Here's how the part is built. I have some questions about the finished solid (model axes, mm). Round coordinates to 2 decimals unless told otherwise and drop trailing zeros. Write each loop counter-clockwise with the first axis right and the second up, starting at its lowest first coordinate (ties: lowest second). Pieces come first, ordered by that corner, then holes. Notation, with made-up numbers: (69, 1) - (102, 1) arc R9 ccw to (102, 15) - close; hole circle Ø1 at (60, -4.5). An arc over 180 degrees is marked (long way). One line per item, written item: value. Start each with the question number.
Item 1: Imagine slicing it at C-C, the plane y = -20. Please give me the cut outline in (x, z), then the cut area to 3 significant figures.
Item 2: Imagine slicing it at B-B, the plane x = 8.5. Please give me the cut outline in (y, z), then the cut area to 3 significant figures.
Item 3: If I drill on line 1 (X direction, y = 63.5, z = -0.1); line 2 (Y direction, x = -1, z = 0.1); line 3 (X direction, y = 31, z = 0.55), over which ranges is the centre line in solid material (lowest first)?
Item 4: Imagine slicing it at A-A, the plane z = 0. Please give me the cut outline in (x, y), then the cut area to 3 significant figures.
Item 5: For P1, Ø1.5, axis at x = 14.5, y = 19, coming from the -Z side; P2, Ø1, axis at x = 0.5, z = 1, coming from the -Y side, each with a flat end and sliding along its axis, tell me the tip position at first contact or that it passes through.
```python
from build123d import *

# Parameters (mm, degrees)
SKETCH5_R = 1.5


with BuildPart() as part:
    # Sweep2: sweep along a path in Sketch4
    with BuildLine(Plane.XY) as sweep2_path:
        Line((-23.236021708, 65.358068893), (-23.236021708, -37.641931107))
        ThreePointArc((-23.236021708, -37.641931107), (-18.549730207, -48.955639606), (-7.236021708, -53.641931107))
        Line((-7.236021708, -53.641931107), (12.563978292, -53.641931107))
        ThreePointArc((12.563978292, -53.641931107), (16.806618979, -51.884571794), (18.563978292, -47.641931107))
        Line((18.563978292, -47.641931107), (18.563978292, 65.358068893))
        ThreePointArc((18.563978292, 65.358068893), (16.806618979, 69.60070958), (12.563978292, 71.358068893))
        Line((12.563978292, 71.358068893), (-17.236021708, 71.358068893))
        ThreePointArc((-17.236021708, 71.358068893), (-21.478662395, 69.60070958), (-23.236021708, 65.358068893))
    # Sketch5 → Sweep2 (sweep)
    with BuildSketch(Plane(origin=(0, 0, 0), x_dir=(1, 0, 0), z_dir=(0, 1, 0))):
        with Locations((-23.236021708, 0)):
            Circle(SKETCH5_R)
    sweep(path=sweep2_path.line)


solid = part.part
```
Values follow:
1. outline: circle Ø3 at (-23.24, 0); circle Ø3 at (18.56, 0)
1. area: 14.1 mm^2
2. outline: circle Ø3 at (-53.64, 0); circle Ø3 at (71.36, 0)
2. area: 14.1 mm^2
3. line 1: x = -24.73 to -21.74, 17.07 to 20.06
3. line 2: y = -55.14 to -52.15, 69.86 to 72.85
3. line 3: x = -24.63 to -21.84, 17.17 to 19.96
4. outline: (-24.74, -37.64) arc R17.5 ccw to (-7.24, -55.14) - (12.56, -55.14) arc R7.5 ccw to (20.06, -47.64) - (20.06, 65.36) arc R7.5 ccw to (12.56, 72.86) - (-17.24, 72.86) arc R7.5 ccw to (-24.74, 65.36) - close; hole (-21.74, -37.64) arc R14.5 ccw to (-7.24, -52.14) - (12.56, -52.14) arc R4.5 ccw to (17.06, -47.64) - (17.06, 65.36) arc R4.5 ccw to (12.56, 69.86) - (-17.24, 69.86) arc R4.5 ccw to (-21.74, 65.36) - close
4. area: 957 mm^2
5. P1: passes through
5. P2: stops at y = -55.06
